from build123d import *

# Parameters (mm, degrees)
SKETCH1_R           = 27.5
SKETCH1_R_2         = 2.0193
SKETCH1_R_3         = 16
BOSS_EXTRUDE1_DEPTH = 5.05
SKETCH2_R           = 38.1
SKETCH2_R_2         = 2.0193
SKETCH2_R_3         = 14
SKETCH2_R_4         = 2.5
BOSS_EXTRUDE2_DEPTH = 2.5
SKETCH3_R           = 25
SKETCH3_R_2         = 17.5
CUT_EXTRUDE1_DEPTH  = 5.05
CHAMFER1_SIZE       = 1


with BuildPart() as part:
    # Sketch1 → Boss-Extrude1 (new body)
    with BuildSketch(Plane(origin=(0, 0, 0), x_dir=(0, 0, -1), z_dir=(1, 0, 0))):
        Circle(SKETCH1_R)
        with Locations((0, 20.64)):
            Circle(SKETCH1_R_2, mode=Mode.SUBTRACT)
        with Locations((17.874764334, 10.32)):
            Circle(SKETCH1_R_2, mode=Mode.SUBTRACT)
        with Locations((17.874764334, -10.32)):
            Circle(SKETCH1_R_2, mode=Mode.SUBTRACT)
        with Locations((0, -20.64)):
            Circle(SKETCH1_R_2, mode=Mode.SUBTRACT)
        with Locations((-17.874764334, -10.32)):
            Circle(SKETCH1_R_2, mode=Mode.SUBTRACT)
        with Locations((-17.874764334, 10.32)):
            Circle(SKETCH1_R_2, mode=Mode.SUBTRACT)
        Circle(SKETCH1_R_3, mode=Mode.SUBTRACT)
    extrude(amount=BOSS_EXTRUDE1_DEPTH)

    # Sketch2 → Boss-Extrude2 (add)
    with BuildSketch(Plane(origin=(5.05, 0, 0), x_dir=(0, 0, -1), z_dir=(1, 0, 0))):
        Circle(SKETCH2_R)
        with Locations((0, 20.64)):
            Circle(SKETCH2_R_2, mode=Mode.SUBTRACT)
        Circle(SKETCH2_R_3, mode=Mode.SUBTRACT)
        with Locations((17.874764334, 10.32)):
            Circle(SKETCH2_R_2, mode=Mode.SUBTRACT)
        with Locations((17.874764334, -10.32)):
            Circle(SKETCH2_R_2, mode=Mode.SUBTRACT)
        with Locations((0, -20.64)):
            Circle(SKETCH2_R_2, mode=Mode.SUBTRACT)
        with Locations((-17.874764334, -10.32)):
            Circle(SKETCH2_R_2, mode=Mode.SUBTRACT)
        with Locations((-17.874764334, 10.32)):
            Circle(SKETCH2_R_2, mode=Mode.SUBTRACT)
        with Locations((0, 32.64)):
            Circle(SKETCH2_R_4, mode=Mode.SUBTRACT)
        with Locations((28.26706918, 16.32)):
            Circle(SKETCH2_R_4, mode=Mode.SUBTRACT)
        with Locations((28.26706918, -16.32)):
            Circle(SKETCH2_R_4, mode=Mode.SUBTRACT)
        with Locations((0, -32.64)):
            Circle(SKETCH2_R_4, mode=Mode.SUBTRACT)
        with Locations((-28.26706918, -16.32)):
            Circle(SKETCH2_R_4, mode=Mode.SUBTRACT)
        with Locations((-28.26706918, 16.32)):
            Circle(SKETCH2_R_4, mode=Mode.SUBTRACT)
    extrude(amount=BOSS_EXTRUDE2_DEPTH)

    # Sketch3 → Cut-Extrude1 (cut)
    with BuildSketch(Plane(origin=(7.55, 0, 0), x_dir=(0, 0, -1), z_dir=(1, 0, 0))):
        Circle(SKETCH3_R)
        Circle(SKETCH3_R_2, mode=Mode.SUBTRACT)
    extrude(amount=-CUT_EXTRUDE1_DEPTH, mode=Mode.SUBTRACT)

    # Chamfer1
    chamfer1_edges = [part.edges().sort_by_distance(p)[0] for p in [
        (5.05, 0, 27.5),
        (7.55, 0, 25),
        (7.55, 0, 17.5),
        (0, 0, 16),
    ]]
    chamfer(chamfer1_edges, length=CHAMFER1_SIZE)


solid = part.part
Geometry: final body of the model. Coordinates: model frame, mm. A direction names the side the tool comes from. Round coordinates to 2 decimals unless told otherwise and drop trailing zeros. Loops run counter-clockwise (first coordinate to the right, second up) from the corner with the lowest first, then second, coordinate; pieces in that order, holes last.
Q1. Section B-B on z = 0. State how many separate pieces and enclosed holes the cut face has, plus the area to 3 significant figures.
Q2. Material intervals for L1, parallel to Y at x = 5.75, z = 0; L2, parallel to Z at x = 5.25, y = -32.5; L3, parallel to Y at x = 4.75, z = -3, sorted ascending.
Q3. Section A-A on y = -32.64. Return loops of the section in (x, z).
Q4. Pull-direction query (Y, two-part tool) for faces 1 (the flat face through (7.55, -12.1, 7.4)), 2 (the cylindrical face through (1.997, -26.846, 5.961)), 3 (the flat face through (5.05, -14.15, 0.07)); classes: released by +Y, released by -Y, zero draft, split by the parting line, or undercut.
Q5. Access query for faces 4 (the cylindrical face through (6.28, 30.2, 0.54)), 5 (the cylindrical face through (3, -15.62, 3.47)). Directions: +Z, -Z, +X, -X, +Y, -Y. A direction counts if a zero-diameter tool reaches every point of the face in a straight line with its end or side. Return the directions, or none.
Q6. Pin query (flat end, axial travel): P1, Ø1.5, axis at x = 3, y = 10, coming from the +Z side; P2, Ø1, axis at x = 1, z = 1, coming from the -Y side; P3, Ø1, axis at x = 6, z = -29.5, coming from the +Y side. Return the tip coordinate at first contact, or that it passes through.
Evaluation:
1. separate pieces: 6
1. enclosed holes: 0
1. area: 114 mm2
2. L1: y = -38.1 to -35.14, -30.14 to -25, -17.5 to -14, 14 to 17.5, 25 to 30.14, 35.14 to 38.1
2. L2: z = -19.88 to -2.5, 2.5 to 19.88
2. L3: y = -28.04 to -24.82, -17.24 to -15.72, 15.72 to 17.24, 24.82 to 28.04
3. outline: (5.05, -19.65) - (7.55, -19.65) - (7.55, -2.5) - (5.05, -2.5) - close; (5.05, 2.5) - (7.55, 2.5) - (7.55, 19.65) - (5.05, 19.65) - close
4. face 1: zero draft
4. face 2: split by the parting line
4. face 3: undercut
5. face 4: +X, -X
5. face 5: -X
6. P1: stops at z = 25.9
6. P2: stops at y = -27.5
6. P3: stops at y = 24.71
